Geometry: final body of the model. Coordinates: model frame, mm. Face numbers are marked on the shaded views. A direction names the side the tool comes from. Round coordinates to 2 decimals unless told otherwise and drop trailing zeros. Write each loop counter-clockwise with the first axis right and the second up, starting at its lowest first coordinate (ties: lowest second). Pieces come first, ordered by that corner, then holes. Notation, with made-up numbers: (-31.75, 85.5) - (25.25, 85.5) arc R11 cw to (25.25, 103.5) - close; hole circle Ø7 at (60.25, 86). An arc over 180 degrees is marked (long way). Write each question's results on one line, items separated by ' | '.
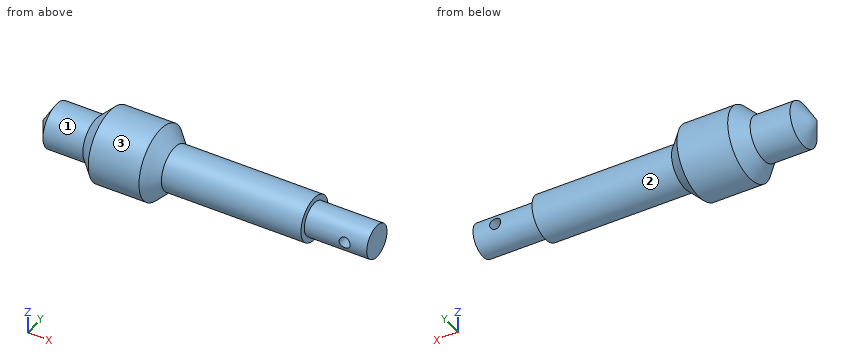
Autodesk Inventor part; units mm, degrees
ref_plane "Work Plane1" through (48.5534, 2.3813, 0) normal (0, 1, 0) x (-1, 0, 0)
ref_plane "YZ Plane" through (0, 0, 0) normal (1, 0, 0) x (0, 1, 0)
ref_plane "XY Plane" through (0, 0, 0) normal (0, 0, 1) x (1, 0, 0)
sketch "Sketch1" plane through (0, 0, 0) normal (0, 0, 1) x (1, 0, 0)
  line L0 (51.1505, 3.175) -> (28.5454, 3.175)
  line L1 (19.2722, 5.1753) -> (17.272, 3.175)
  line L2 (26.5452, 5.1753) -> (28.5454, 3.175)
  line L3 (9.6514, 0) -> (11.5592, 3.175)
  line L4 (17.272, 3.175) -> (11.5592, 3.175)
  line L5 (26.5452, 5.1753) -> (19.2722, 5.1753)
  line L6 (9.6514, 0) -> (51.1505, 0)
  line L7 (51.1505, 3.175) -> (51.1505, 0)
  point P0 (0, 0)
  dimension "d3" = 135
  dimension "d4" = 7.2729
  dimension "d5" = 5.7128
  dimension "d8" = 59
  dimension "d9" = 135
  dimension "d10" = 41.4991
  dimension "d11" = 3.175
  dimension "d12" = 5.1753
  dimension "d13" = 3.175
  dimension "d14" = 9.6514
revolve "Revolution1" add sketch "Sketch1" angle 360 about axis through (9.6514, 0, 0) along (1, 0, 0)
sketch "Sketch2" plane through (51.1505, 0, 0) normal (1, 0, 0) x (0, 0, -1)
  circle A0 centre (0, 0) radius 3.175
extrude "Extrusion1" cut sketch "Sketch2" against normal blind 4.9784
sketch "Sketch5" plane through (46.1721, 0, 0) normal (1, 0, 0) x (0, 0, -1)
  circle A0 centre (0, 0) radius 3.175
extrude "Extrusion4" add sketch "Sketch5" along normal blind 2.3813
sketch "Sketch6" plane through (48.5534, 0, 0) normal (1, 0, 0) x (0, 0, -1)
  circle A0 centre (0, 0) radius 3.175
  circle A1 centre (0, 0) radius 2.3813
  dimension "d30" = 4.7625
extrude "Extrusion5" add sketch "Sketch6" along normal blind 8.9472 contours A1
ref_plane "Work Plane1" through (48.5534, 2.3813, 0) normal (0, 1, 0) x (-1, 0, 0)
sketch "Sketch7" plane through (48.5534, 2.3813, 0) normal (0, 1, 0) x (-1, 0, 0)
  line L0 (-8.9471, 2.3813) -> (-8.9471, -2.3813)
  line L1 (0, -2.3813) -> (0, 2.3813)
  line L2 (-8.9471, 0) -> (0, 0) construction
  circle A0 centre (-5.7721, 0) radius 0.7937
  point P0 (48.5534, 0)
  dimension "d34" = 1.5875
  dimension "d36" = 5.7721
extrude "Extrusion6" cut sketch "Sketch7" against normal through all
properties part number "Ball Shifting Shaft" material "Steel"
Q1. Pin query (flat end, axial travel): pin 1 (1.5 mm diameter, centred on x = 51.5, y = -0.5, fed in from -Z); pin 2 (6 mm diameter, centred on x = 52.5, z = -0.5, fed in from +Y); pin 3 (1.5 mm diameter, centred on x = 40, z = 0.5, fed in from +Y) (3 decimals); pin 4 (1.3 mm diameter, centred on x = 54.33, z = 0, fed in from +Y). Return the tip coordinate at first contact, or that it passes through.
Answer block:
pin 1: z = -2.38 | pin 2: y = 2.38 | pin 3: y = 3.175 | pin 4: through
Q2. Section query A-A, the plane x = 41.5. Return loops of the section in (y, z) (3 decimals), plus the area to 3 significant figures.
Answer block:
outline: circle Ø6.35 at (0, 0) | area: 31.7 mm2
Q3. Section query B-B, the plane x = 23.5. Return loops of the section in (y, z), plus the area to 3 significant figures.
Answer block:
outline: circle Ø10.35 at (0, 0) | area: 84.1 mm2
Q4. Ray query, line 1 along X through (y, z) = (0.95, 0); line 2 along Z through (x, y) = (45, -0.25); line 3 along X through (y, z) = (-0.55, 0). Return the intervals inside material, ascending.
Answer block:
line 1: 10.22 to 53.53, 55.12 to 57.5 | line 2: -3.17 to 3.17 | line 3: 9.98 to 53.53, 55.12 to 57.5
Q5. Access query for the marked faces 1, 2 and 3. Directions: +Z, -Z, +X, -X, +Y, -Y. A direction counts if a zero-diameter tool reaches every point of the face in a straight line with its end or side. Return the directions, or none.
Answer block:
face 1: -X | face 2: +X | face 3: +X, -X
